```python
from build123d import *

# Parameters (mm, degrees)
SKETCH1_W           = 50.2
SKETCH1_H           = 9.92
SKETCH1_R           = 1.65
BOSS_EXTRUDE1_DEPTH = 1.32
SKETCH2_R           = 4.575
BOSS_EXTRUDE2_DEPTH = 6.5
SKETCH3_R           = 0.75
CUT_EXTRUDE1_DEPTH  = 1.5
SKETCH4_W           = 4.85
SKETCH4_H           = 4.85
BOSS_EXTRUDE3_DEPTH = 1.6


with BuildPart() as part:
    # Sketch1 → Boss-Extrude1 (new body)
    with BuildSketch(Plane(origin=(0, 0, 0), x_dir=(1, 0, 0), z_dir=(0, 1, 0))):
        Rectangle(SKETCH1_W, SKETCH1_H)
        with Locations(Location((-15.25, -2.66, 0), (0, 0, 270))):
            Circle(SKETCH1_R, mode=Mode.SUBTRACT)
        with Locations(Location((15.25, -2.66, 0), (0, 0, 90))):
            Circle(SKETCH1_R, mode=Mode.SUBTRACT)
    extrude(amount=BOSS_EXTRUDE1_DEPTH)

    # Sketch2 → Boss-Extrude2 (add)
    with BuildSketch(Plane(origin=(0, 1.32, 0), x_dir=(1, 0, 0), z_dir=(0, 1, 0))):
        with Locations(Location((0, 0, 0), (0, 0, 90))):
            Circle(SKETCH2_R)
    extrude(amount=BOSS_EXTRUDE2_DEPTH)

    # Sketch3 → Cut-Extrude1 (cut)
    with BuildSketch(Plane(origin=(0, 7.82, 0), x_dir=(1, 0, 0), z_dir=(0, 1, 0))):
        with Locations(Location((0, 0, 0), (0, 0, 270))):
            Circle(SKETCH3_R)
    extrude(amount=-CUT_EXTRUDE1_DEPTH, mode=Mode.SUBTRACT)

    # Sketch4 → Boss-Extrude3 (add)
    with BuildSketch(Plane(origin=(0, 1.32, 0), x_dir=(1, 0, 0), z_dir=(0, 1, 0))):
        with Locations((-8.6, 1.76)):
            Rectangle(SKETCH4_W, SKETCH4_H)
        with Locations((-15.1, 1.76)):
            Rectangle(SKETCH4_W, SKETCH4_H)
        with Locations((-21.6, 1.76)):
            Rectangle(SKETCH4_W, SKETCH4_H)
        with Locations((8.6, 1.76)):
            Rectangle(SKETCH4_W, SKETCH4_H)
        with Locations((15.1, 1.76)):
            Rectangle(SKETCH4_W, SKETCH4_H)
        with Locations((21.6, 1.76)):
            Rectangle(SKETCH4_W, SKETCH4_H)
    extrude(amount=BOSS_EXTRUDE3_DEPTH)


solid = part.part
```
Design review of the part built by this model. Coordinates are the model's own, in mm. A direction names the side the tool comes from. Coordinates: 2 decimals unless noted, no trailing zeros. Loops run counter-clockwise (first coordinate to the right, second up) from the corner with the lowest first, then second, coordinate; pieces in that order, holes last.
Q1. We need section A-A on x = 15.25. State the section outline as (y, z) points (3 decimals), and give its area (3 significant figures).
Reported:
outline: (0, -4.96) - (1.32, -4.96) - (1.32, -4.185) - (2.92, -4.185) - (2.92, 0.665) - (1.32, 0.665) - (1.32, 1.01) - (0, 1.01) - close; (0, 4.31) - (1.32, 4.31) - (1.32, 4.96) - (0, 4.96) - close
area: 16.5 mm2
Q2. We need section B-B on y = 2.5. State the section outline as (x, z) points (3 decimals), and give its area (3 significant figures).
Reported:
outline: (-24.025, -4.185) - (-19.175, -4.185) - (-19.175, 0.665) - (-24.025, 0.665) - close; (-17.525, -4.185) - (-12.675, -4.185) - (-12.675, 0.665) - (-17.525, 0.665) - close; (-11.025, -4.185) - (-6.175, -4.185) - (-6.175, 0.665) - (-11.025, 0.665) - close; circle Ø9.15 at (0, 0); (6.175, -4.185) - (11.025, -4.185) - (11.025, 0.665) - (6.175, 0.665) - close; (12.675, -4.185) - (17.525, -4.185) - (17.525, 0.665) - (12.675, 0.665) - close; (19.175, -4.185) - (24.025, -4.185) - (24.025, 0.665) - (19.175, 0.665) - close
area: 207 mm2
Q3. We need section C-C on z = 3.5. State the section outline as (x, y) points, and give its area (3 significant figures).
Reported:
outline: (-25.1, 0) - (-16.67, 0) - (-16.67, 1.32) - (-25.1, 1.32) - close; (-13.83, 0) - (13.83, 0) - (13.83, 1.32) - (2.95, 1.32) - (2.95, 7.82) - (-2.95, 7.82) - (-2.95, 1.32) - (-13.83, 1.32) - close; (16.67, 0) - (25.1, 0) - (25.1, 1.32) - (16.67, 1.32) - close
area: 97.1 mm2
Q4. Tool access review of faces 1 (the face through (-15, 2, -4.185)), 2 (the face through (-15, 2, 0.665)), 3 (the face through (15, 2, -4.185)), 4 (the face through (-12.675, 2, -2)): name each direction out of +Z, -Z, +X, -X, +Y, -Y from which nothing blocks a thin tool from reaching the whole face with its end or side.
Reported:
face 1: -Z, -X, +Y
face 2: +Z, -X, +Y
face 3: -Z, +X, +Y
face 4: +Z, -Z, +Y
Q5. For pin 1 (1.6 mm diameter, centred on x = 0, z = 0.5, fed in from +Y); pin 2 (1.3 mm diameter, centred on y = 2, z = -2, fed in from +X) (3 decimals); pin 3 (1.8 mm diameter, centred on x = -22.5, y = 2.5, fed in from -Z) (3 decimals); pin 4 (5.5 mm diameter, centred on x = 9, z = -1, fed in from +Y), all flat-tipped, find the tip position at first contact; note any pin that passes through.
Reported:
pin 1: stops at y = 7.82
pin 2: stops at x = 24.025
pin 3: stops at z = -4.185
pin 4: stops at y = 2.92
Q6. We need section D-D on x = 20.5. State the section outline as (y, z) points (3 decimals), and give its area (3 significant figures).
Reported:
outline: (0, -4.96) - (1.32, -4.96) - (1.32, -4.185) - (2.92, -4.185) - (2.92, 0.665) - (1.32, 0.665) - (1.32, 4.96) - (0, 4.96) - close
area: 20.9 mm2
Q7. The part is to be moulded in two halves that separate along X. For faces 5 (the face through (24.025, 2, -2)), 6 (the face through (17.525, 2, -2)), 7 (the face through (-9, 2.92, -2)), say which applies: +X half, -X half, draft (parallel to the pull), parting line (faces both ways), or undercut.
Reported:
face 5: +X half
face 6: undercut
face 7: draft
Q8. To check wall thickness, follow line 1 (X direction, y = 0.3, z = 2.66); line 2 (X direction, y = 7.35, z = 0) (3 decimals); line 3 (Y direction, x = -22, z = -0.25). State the ranges of each line that lie inside material, in increasing order.
Reported:
line 1: x = -25.1 to -16.9, -13.6 to 13.6, 16.9 to 25.1
line 2: x = -4.575 to -0.75, 0.75 to 4.575
line 3: y = 0 to 2.92
